The drawing under review shows one solid part. Ordinate dimensions are in mm from its lowest x, y, z. Coordinates: 2 decimals unless noted, no trailing zeros. Write each loop counter-clockwise with the first axis right and the second up, starting at its lowest first coordinate (ties: lowest second). Pieces come first, ordered by that corner, then holes.
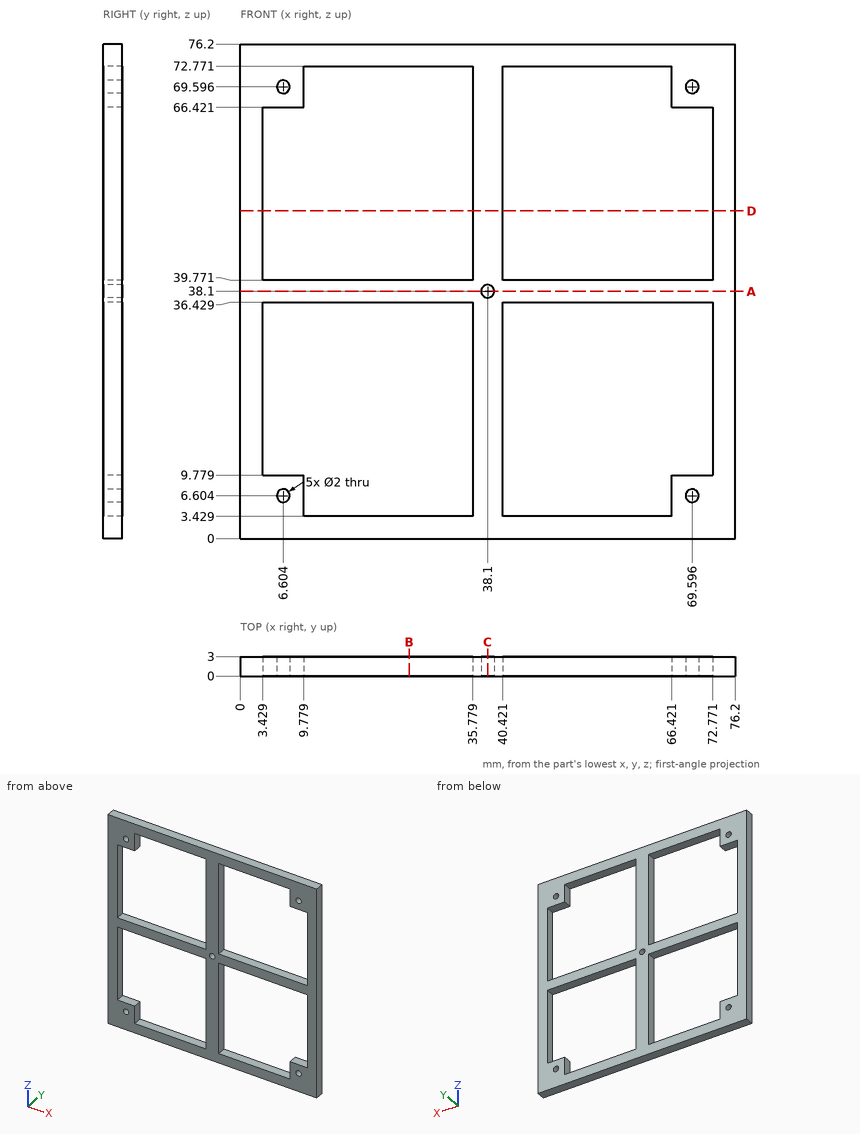
Q1. Add section A-A (z = 38.1). State the section outline as (x, y) points, then the cut area to 3 significant figures.
Ans:
outline: (0, 0) - (37.1, 0) - (37.1, 3) - (0, 3) - close; (39.1, 0) - (76.2, 0) - (76.2, 3) - (39.1, 3) - close
area: 223 mm2
Q2. Add section C-C (x = 38.1). State the section outline as (y, z) points.
Ans:
outline: (0, 0) - (3, 0) - (3, 37.1) - (0, 37.1) - close; (0, 39.1) - (3, 39.1) - (3, 76.2) - (0, 76.2) - close
Q3. For probe 1 along X at (y, z) = (2, 14); probe 2 along Z at (x, y) = (13.5, 1.55); probe 3 along Z at (x, y) = (68, 0.75), list the stretches that pass through material, from the lowest coordinate up.
Ans:
probe 1: x = 0 to 3.43, 35.78 to 40.42, 72.77 to 76.2
probe 2: z = 0 to 3.43, 36.43 to 39.77, 72.77 to 76.2
probe 3: z = 0 to 9.78, 36.43 to 39.77, 66.42 to 76.2
Q4. Add section D-D (z = 50.5). State the section outline as (x, y) points, then the cut area to 3 significant figures.
Ans:
outline: (0, 0) - (3.43, 0) - (3.43, 3) - (0, 3) - close; (35.78, 0) - (40.42, 0) - (40.42, 3) - (35.78, 3) - close; (72.77, 0) - (76.2, 0) - (76.2, 3) - (72.77, 3) - close
area: 34.5 mm2
Q5. Add section B-B (x = 26). State the section outline as (y, z) points, then the cut area to 3 significant figures.
Ans:
outline: (0, 0) - (3, 0) - (3, 3.43) - (0, 3.43) - close; (0, 36.43) - (3, 36.43) - (3, 39.77) - (0, 39.77) - close; (0, 72.77) - (3, 72.77) - (3, 76.2) - (0, 76.2) - close
area: 30.6 mm2
